Source: three-view drawing plus pictorial views. Frame: mm from the lowest corner of the part. Round coordinates to 2 decimals unless told otherwise and drop trailing zeros. Order: outer loops, then holes, each group sorted by start corner. A loop starts at its lowest first (then second) coordinate and runs counter-clockwise, first axis right, second up. Notation, with made-up numbers: (28, -23.75) -> (35, -23.75) arc R15 cw to (35, -0.75) -> close; hole circle Ø1 at (-8.5, 88.5). An arc over 180 degrees is marked (long way). Answer as CSV lines item,"result".
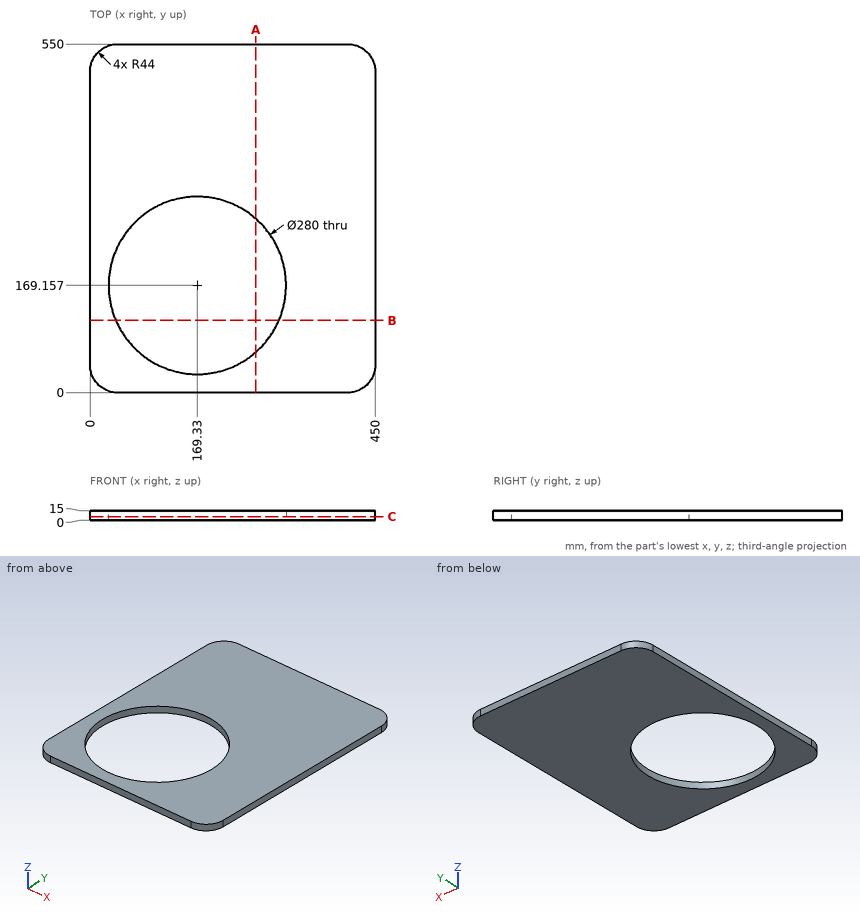
1. Line query: L1, parallel to X at y = 269, z = 8.5; L2, parallel to Y at x = 208.5, z = 1.5 (1 decimal); L3, parallel to Y at x = 255.5, z = 8.25 (1 decimal). Output: solid intervals per line, ascending. Write a range as [from, to].
Results below:
L1,"[0, 71.19], [267.47, 450]"
L2,"[0, 34.7], [303.6, 550]"
L3,"[0, 58.8], [279.5, 550]"
2. Section query A-A on x = 261.5. Return loops of the section in (y, z) (1 decimal).
Results below:
outline,"(0, 0) -> (63.8, 0) -> (63.8, 15) -> (0, 15) -> close; (274.5, 0) -> (550, 0) -> (550, 15) -> (274.5, 15) -> close"
3. Section query C-C on z = 5.5. Return loops of the section in (x, y).
Results below:
outline,"(0, 44) arc R44 ccw to (44, 0) -> (406, 0) arc R44 ccw to (450, 44) -> (450, 506) arc R44 ccw to (406, 550) -> (44, 550) arc R44 ccw to (0, 506) -> close; hole circle Ø280 at (169.33, 169.16)"
4. Section query B-B on y = 114. Return loops of the section in (x, z), and give its area (3 significant figures).
Results below:
outline,"(0, 0) -> (40.65, 0) -> (40.65, 15) -> (0, 15) -> close; (298.01, 0) -> (450, 0) -> (450, 15) -> (298.01, 15) -> close"
area,"2,890 mm2"
